Work out the finished part from the listing and answer in its coordinate system (mm). A direction names the side the tool comes from. Give positions to 0.01 mm unless a question says otherwise; leave off trailing zeros. Write each loop counter-clockwise with the first axis right and the second up, starting at its lowest first coordinate (ties: lowest second). Pieces come first, ordered by that corner, then holes. Notation, with made-up numbers: (14, 15.5) - (71, 15.5) arc R28 ccw to (71, 42.5) - close; hole circle Ø3 at (-37.75, 35). An arc over 180 degrees is marked (long way). Write item = value, one per line.
from build123d import *

# Parameters (mm, degrees)
BOSS_EXTRUDE1_DEPTH = 76.2
CUT_EXTRUDE1_DEPTH  = 19.05
CUT_EXTRUDE2_DEPTH  = 19.05
SKETCH4_R           = 3.175
CUT_EXTRUDE3_DEPTH  = 13.7


with BuildPart() as part:
    # Sketch1 → Boss-Extrude1 (new body)
    with BuildSketch(Plane.XY):
        with BuildLine():
            Line((-6.35, -12.7), (6.35, -12.7))
            add(Edge.make_bspline(
                [(6.35, 12.7), (25.715251748, 11.504486328), (-0.315251748, 0), (25.715251748, -11.504486328), (6.35, -12.7)],
                knots=[0, 0, 0, 0, 0.5, 1, 1, 1, 1], degree=3))
            Line((6.35, 12.7), (-6.35, 12.7))
            Line((-6.35, 12.7), (-6.35, -12.7))
        make_face()
    extrude(amount=BOSS_EXTRUDE1_DEPTH)

    # Sketch2 → Cut-Extrude1 (cut)
    with BuildSketch(Plane.XY.offset(76.2)):
        with BuildLine():
            Line((6.35, 12.7), (6.35, -12.7))
            add(Edge.make_bspline(
                [(6.35, -12.7), (25.715251748, -11.504486328), (-0.315251748, 0), (25.715251748, 11.504486328), (6.35, 12.7)],
                knots=[0, 0, 0, 0, 0.5, 1, 1, 1, 1], degree=3))
        make_face()
    extrude(amount=-CUT_EXTRUDE1_DEPTH, mode=Mode.SUBTRACT)

    # Sketch3 → Cut-Extrude2 (cut)
    with BuildSketch(Plane(origin=(0, 0, 0), x_dir=(-1, 0, 0), z_dir=(0, 0, -1))):
        with BuildLine():
            Line((-6.35, 12.7), (-6.35, -12.7))
            add(Edge.make_bspline(
                [(-6.35, -12.7), (-25.715251748, -11.504486328), (0.315251748, 0), (-25.715251748, 11.504486328), (-6.35, 12.7)],
                knots=[0, 0, 0, 0, 0.5, 1, 1, 1, 1], degree=3))
        make_face()
    extrude(amount=-CUT_EXTRUDE2_DEPTH, mode=Mode.SUBTRACT)

    # Sketch4 → Cut-Extrude3 (cut, through all)
    with BuildSketch(Plane(origin=(6.35, 0, 0), x_dir=(0, 0, -1), z_dir=(1, 0, 0))):
        with Locations((-66.675, 0)):
            Circle(SKETCH4_R)
        with Locations((-9.525, 0)):
            Circle(SKETCH4_R)
    extrude(amount=-CUT_EXTRUDE3_DEPTH, mode=Mode.SUBTRACT)


solid = part.part
1. Find section B-B, the plane y = 0. Give the number of separate pieces and of enclosed holes in the cut face, then the cut area to 3 significant figures.
Solution:
separate_pieces = 3
enclosed_holes = 0
area = 1,050 mm^2
2. For a pull along Y with two mould halves and no side action, classify faces 1 (the flat face through (0, 12.7, 38)), 2 (the cylindrical face through (0.089, -1.932, 12.045)), 3 (the cylindrical face through (0.089, 0.954, 63.647)), 4 (the flat face through (6.35, -3, 65)) as pulls with the +Y half, pulls with the -Y half, needs draft (parallel to the pull), parting line crosses it, or undercut.
Solution:
face_1 = pulls with the +Y half
face_2 = undercut
face_3 = undercut
face_4 = needs draft
3. Find section A-A, the plane x = -0.5. Give the vertices of the cut face in (y, z) (3 decimals), then the cut area to 3 significant figures.
Solution:
outline = (-12.7, 0) - (12.7, 0) - (12.7, 76.2) - (-12.7, 76.2) - close; hole circle Ø6.35 at (0, 9.525); hole circle Ø6.35 at (0, 66.675)
area = 1,870 mm^2
4. Given pin 1 (3 mm diameter, centred on x = 11, y = 2.5, fed in from +Z); pin 2 (1.5 mm diameter, centred on y = 5, z = 26.5, fed in from +X); pin 3 (1.5 mm diameter, centred on x = 13, z = 19.5, fed in from -Y), each flat-ended and moving along its own axis, determine where each tip first touches the part or whether it passes through.
Solution:
pin_1 = 57.15
pin_2 = 15.47
pin_3 = -12.03
5. Straight lines are drawn through the part: line 1 (Z direction, x = 11.25, y = -4.25); line 2 (X direction, y = -3.75, z = 64); line 3 (Y direction, x = 15.5, z = 26.5). For each, find the intervals that lie inside material, in ascending order.
Solution:
line_1 = 19.05 to 57.15
line_2 = -6.35 to 6.35
line_3 = -11.03 to -5.79, 5.79 to 11.03
6. A tool of negligible diameter and unlimited length cuts with its end or side. For faces 5 (the flat face through (10, 0, 19.05)), 6 (the flat face through (10, 0, 57.15)), 7 (the flat face through (0, 0, 0)), from which of +Z, -Z, +X, -X, +Y, -Y can it reach the whole face along a straight path? Write none if from no direction.
Solution:
face_5 = -Z, +X, +Y, -Y
face_6 = +Z, +X, +Y, -Y
face_7 = -Z, +X, -X, +Y, -Y
